```python
from build123d import *

# Parameters (mm, degrees)
SKETCH1_W                             = 8
SKETCH1_H                             = 3.8
BE_01_BOSS_EXTRUDE_DEPTH              = 2.5
CE_01_CLAMP_GROOVES_DEPTH             = 3
F_52_0_0635_DIAMETER_HOLE1_AT_2_COUNT = 2
F_52_0_0635_DIAMETER_HOLE1_AT_2_PITCH = 4.2
FILLET1_R                             = 0.4


with BuildPart() as part:
    # Sketch1 → BE-01 Boss Extrude (new body)
    with BuildSketch(Plane(origin=(0, 0, 0), x_dir=(1, 0, 0), z_dir=(0, 1, 0))):
        Rectangle(SKETCH1_W, SKETCH1_H)
    extrude(amount=BE_01_BOSS_EXTRUDE_DEPTH)

    # Sketch2 → CE-01 Clamp Grooves (cut, symmetric)
    with BuildSketch(Plane.XY):
        with BuildLine():
            Line((-6.978653293, -2.49), (-6.978653293, -4.211330321))
            Line((-6.978653293, -4.211330321), (6.978653293, -4.211330321))
            Line((6.978653293, -4.211330321), (6.978653293, -2.49))
            Line((6.978653293, -2.49), (1.0668, -2.49))
            Line((1.0668, -2.49), (1.0668, 0.05))
            ThreePointArc((1.0668, 0.05), (0.635, 0.4818), (0.2032, 0.05))
            Line((0.2032, 0.05), (0.2032, -2.49))
            Line((0.2032, -2.49), (-0.2032, -2.49))
            Line((-0.2032, -2.49), (-0.2032, 0.05))
            ThreePointArc((-0.2032, 0.05), (-0.635, 0.4818), (-1.0668, 0.05))
            Line((-1.0668, 0.05), (-1.0668, -2.49))
            Line((-1.0668, -2.49), (-6.978653293, -2.49))
        make_face()
    extrude(amount=CE_01_CLAMP_GROOVES_DEPTH, both=True, mode=Mode.SUBTRACT)

    # Sketch4 → #52 (0.0635) Diameter Hole1 (revolve, cut)
    with BuildSketch(Plane(origin=(-2.1, 2.5, 0), x_dir=(0, 0, 1), z_dir=(1, 0, 0))):
        Polygon((0, 0), (0, 2.5), (0.8636, 2.5), (0.80645, 2.44285), (0.80645, 0.05715), (0.8636, 0), align=None)
    f_52_0_0635_diameter_hole1 = revolve(axis=Axis((-2.1, 8.85, 0), (0, -1, 0)), mode=Mode.SUBTRACT)

    # #52 (0.0635) Diameter Hole1 at 2: #52 (0.0635) Diameter Hole1 ×2
    with Locations(*[(i * F_52_0_0635_DIAMETER_HOLE1_AT_2_PITCH, 0, 0) for i in range(1, F_52_0_0635_DIAMETER_HOLE1_AT_2_COUNT)]):
        add(f_52_0_0635_diameter_hole1, mode=Mode.SUBTRACT)

    # Fillet1
    fillet1_edges = [part.edges().sort_by_distance(p)[0] for p in [
        (-4, 1.25, -1.9),
        (4, 1.25, -1.9),
        (4, 1.25, 1.9),
        (-4, 1.25, 1.9),
    ]]
    fillet(fillet1_edges, radius=FILLET1_R)


solid = part.part
```
Here's how the part is built. I have some questions about the finished solid (model axes, mm). Round coordinates to 2 decimals unless told otherwise and drop trailing zeros. Order: outer loops, then holes, each group sorted by start corner. A loop starts at its lowest first (then second) coordinate and runs counter-clockwise, first axis right, second up. Notation, with made-up numbers: (49, -5) -> (72, -5) arc R13 cw to (72, 4) -> close; hole circle Ø8 at (20, 27). An arc over 180 degrees is marked (long way). Use a Markdown table: item, result. Add a question column.
(1) Suppose I cut it at C-C, the plane y = 0.7. Please give me the cut outline in (x, z), and give its area (3 significant figures).
(2) Suppose I cut it at B-B, the plane x = -2.1. Please give me the cut outline in (y, z), and give its area (3 significant figures).
(3) If we mould it in two halves opening along X, with no side actions, what happens to faces 1 (the face through (0, 1, 1.9)), 2 (the face through (4, 1, 0)), 3 (the face through (2.8, 1.3, 0.4))? For each: released by +X, released by -X, zero draft, split by the parting line, or undercut.
(4) I need wall thicknesses on line 1 along X through (y, z) = (0.7, 0); line 2 along Z through (x, y) = (-2.1, 1.1); line 3 along X through (y, z) = (1.5, 0.5). Which ranges of each line are inside material? Lowest first, please.
(5) Suppose I cut it at D-D, the plane z = -1. Please give me the cut outline in (x, y) (3 decimals), and give its area (3 significant figures).
(6) Suppose I cut it at A-A, the plane z = 0. Please give me the cut outline in (x, y) (3 decimals), and give its area (3 significant figures).
Verdict:
| question | item | result |
|---|---|---|
| 1 | outline | (-4, -1.5) arc R0.4 ccw to (-3.6, -1.9) -> (3.6, -1.9) arc R0.4 ccw to (4, -1.5) -> (4, 1.5) arc R0.4 ccw to (3.6, 1.9) -> (-3.6, 1.9) arc R0.4 ccw to (-4, 1.5) -> close; hole circle Ø1.61 at (-2.1, 0); hole circle Ø1.61 at (2.1, 0) |
| 1 | area | 26.2 mm2 |
| 2 | outline | (0, -1.9) -> (2.5, -1.9) -> (2.5, -0.86) -> (2.44, -0.81) -> (0.06, -0.81) -> (0, -0.86) -> close; (0, 0.86) -> (0.06, 0.81) -> (2.44, 0.81) -> (2.5, 0.86) -> (2.5, 1.9) -> (0, 1.9) -> close |
| 2 | area | 5.46 mm2 |
| 3 | face 1 | zero draft |
| 3 | face 2 | released by +X |
| 3 | face 3 | undercut |
| 4 | line 1 | -4 to -2.91, -1.29 to 1.29, 2.91 to 4 |
| 4 | line 2 | -1.9 to -0.81, 0.81 to 1.9 |
| 4 | line 3 | -4 to -2.73, -1.47 to 1.47, 2.73 to 4 |
| 5 | outline | (-4, 0) -> (-1.067, 0) -> (-1.067, 0.05) arc R0.432 cw to (-0.203, 0.05) -> (-0.203, 0) -> (0.203, 0) -> (0.203, 0.05) arc R0.432 cw to (1.067, 0.05) -> (1.067, 0) -> (4, 0) -> (4, 2.5) -> (-4, 2.5) -> close |
| 5 | area | 19.3 mm2 |
| 6 | outline | (-4, 0) -> (-2.964, 0) -> (-2.906, 0.057) -> (-2.906, 2.443) -> (-2.964, 2.5) -> (-4, 2.5) -> close; (-1.294, 0.057) -> (-1.236, 0) -> (-1.067, 0) -> (-1.067, 0.05) arc R0.432 cw to (-0.203, 0.05) -> (-0.203, 0) -> (0.203, 0) -> (0.203, 0.05) arc R0.432 cw to (1.067, 0.05) -> (1.067, 0) -> (1.236, 0) -> (1.294, 0.057) -> (1.294, 2.443) -> (1.236, 2.5) -> (-1.236, 2.5) -> (-1.294, 2.443) -> close; (2.906, 0.057) -> (2.964, 0) -> (4, 0) -> (4, 2.5) -> (2.964, 2.5) -> (2.906, 2.443) -> close |
| 6 | area | 11.3 mm2 |
